Source: CAD feature listing. Evaluate the final solid. Frame: model axes, mm. A direction names the side the tool comes from. Coordinates: 2 decimals unless noted, no trailing zeros. Write each loop counter-clockwise with the first axis right and the second up, starting at its lowest first coordinate (ties: lowest second). Pieces come first, ordered by that corner, then holes. Notation, with made-up numbers: M 30.25,24 L 54.25,24 A21 ccw 54.25,31 Z; hole C 29.25,63.25 d1. An arc over 180 degrees is marked long. One line per item, written item: value. Start each with the question number.
Item 1: Ray query, L1, parallel to Z at x = 329, y = -14; L2, parallel to Z at x = 325, y = -7.5; L3, parallel to X at y = -9, z = 167. Return the intervals inside material, ascending. Write a range as from..to.
Item 2: Cut plane C-C, the plane x = -141.5. Output: boundary loops of the cut face in (y, z), then the cut area to 3 significant figures.
Item 3: Cut plane B-B, the plane z = 289. Output: boundary loops of the cut face in (x, y).
Item 4: Mould query, pull axis X, two halves, no side actions, for faces 1 (the flat face through (84, 0, 465)), 2 (the flat face through (342.525, -22.185, 760.85)), 3 (the flat face through (139.112, -22, 285)), 4 (the flat face through (-57, -22, 45)). Classes: released by +X, released by -X, zero draft, split by the parting line, or undercut.
Item 5: Set-up query: faces 5 (the flat face through (593.112, -22, 977)), 6 (the flat face through (-62.3, -22.2, 278.4)), 7 (the flat face through (184.112, -22, 282)), 8 (the flat face through (84, -45, 465)), 9 (the flat face through (139.112, -22, 797)). Return all of +Z, -Z, +X, -X, +Y, -Y with unobstructed straight access to the full face (end or side cutting, diameter ignored); none if empty.
Item 6: Cut plane D-D, the plane x = 484. Output: boundary loops of the cut face in (y, z), then the cut area to 3 significant figures.
Item 7: Cut plane A-A, the plane y = -24.5. Output: boundary loops of the cut face in (x, z).
Item 8: Pin query (flat end, axial travel): P1, Ø8, axis at y = -12.5, z = 813, coming from the +X side; P2, Ø1, axis at x = 247, y = -16.5, coming from the -Z side; P3, Ø1, axis at y = -38, z = 482.5, coming from the -X side. Return the tip coordinate at first contact, or that it passes through.
```python
from build123d import *

# Parameters (mm, degrees)
F0_W     = 45
F0_H     = 45
F1_DEPTH = 45


with BuildPart() as f1:
    # F0 (on Front) → F1 (new body)
    with BuildSketch(Plane.XZ):
        Polygon((139.1122582526, 518.4320460093), (139.1122582526, 588.439618218), (-316.8877249613, 45), (-258.1443969413, 45), align=None)
        Polygon((-258.1443969413, 45), (-316.8877249613, 45), (-351.3597249985, 3.9178701118), (-346.6905892175, 0), (-295.9038803443, 0), align=None)
        Polygon((139.1122582526, 0), (139.1122582526, 45), (-258.1443969413, 45), (-295.9038803443, 0), align=None)
        with Locations((161.6122582526, 22.5)):
            Rectangle(F0_W, F0_H)
        Polygon((184.1122582526, 45), (184.1122582526, 572.060957676), (139.1122582526, 518.4320460093), (139.1122582526, 45), align=None)
        Polygon((184.1122582526, 600), (148.8125703421, 600), (139.1122582526, 588.439618218), (139.1122582526, 518.4320460093), (184.1122582526, 572.060957676), align=None)
        Polygon((184.1122582526, 642.0685298847), (184.1122582526, 600), (184.1122582526, 572.060957676), (505.43626743, 955), (446.6929394101, 955), align=None)
        with Locations((161.6122582526, 977.5)):
            Rectangle(F0_W, F0_H)
        Polygon((184.1122582526, 1000), (184.1122582526, 955), (446.6929394101, 955), (484.264167594, 999.7756461664), (518.7361675344, 970.8502037305), (505.43626743, 955), (593.1122582526, 955), (593.1122582526, 1000), align=None)
        Polygon((139.1122582526, 588.439618218), (148.8125703421, 600), (184.1122582526, 642.0685298847), (184.1122582526, 955), (139.1122582526, 955), align=None)
        Polygon((484.264167594, 999.7756461664), (446.6929394101, 955), (505.43626743, 955), (518.7361675344, 970.8502037305), align=None)
        Polygon((184.1122582526, 642.0685298847), (148.8125703421, 600), (184.1122582526, 600), align=None)
    extrude(amount=F1_DEPTH)


solid = f1.part
```
From the geometry:
1. L1: z = 744.73..814.74, 955..1000
1. L2: z = 739.96..809.97, 955..1000
1. L3: x = -214.52..-155.77, 139.11..184.11
2. outline: M -45,0 L 0,0 L 0,45 L -45,45 Z; M -45,184.01 L 0,184.01 L 0,254.02 L -45,254.02 Z
2. area: 5,180 mm²
3. outline: M -112.15,-45 L -53.4,-45 L -53.4,0 L -112.15,0 Z; M 139.11,-45 L 184.11,-45 L 184.11,0 L 139.11,0 Z
4. face 1: zero draft
4. face 2: released by +X
4. face 3: undercut
4. face 4: undercut
5. face 5: +Z, -Z, +X, +Y, -Y
5. face 6: +Y, -Y
5. face 7: -Z, +X, +Y, -Y
5. face 8: +Z, -Z, +X, -X, -Y
5. face 9: +Z, -X, +Y, -Y
6. outline: M -45,929.45 L 0,929.45 L 0,1000 L -45,1000 Z
6. area: 3,170 mm²
7. outline: M -351.36,3.92 L -346.69,0 L 184.11,0 L 184.11,572.06 L 505.44,955 L 593.11,955 L 593.11,1000 L 139.11,1000 L 139.11,588.44 Z; hole M -258.14,45 L 139.11,45 L 139.11,518.43 Z; hole M 184.11,642.07 L 446.69,955 L 184.11,955 Z
8. P1: stops at x = 389.64
8. P2: stops at z = 646.41
8. P3: stops at x = 49.8
